```python
from build123d import *

# Parameters (mm, degrees)
SKETCH_1_W          = 57.5
SKETCH_1_H          = 46.5
EXTRUDE_1_DEPTH     = 3
SKETCH_2_R          = 1
CUT_EXTRUDE_1_DEPTH = 38.096158831
SKETCH_4_R          = 2.6
CUT_EXTRUDE_2_DEPTH = 0.8


with BuildPart() as part:
    # 草图1 → 凸台-拉伸1 (new body)
    with BuildSketch(Plane(origin=(0, 0, 0), x_dir=(1, 0, 0), z_dir=(0, 1, 0))):
        Rectangle(SKETCH_1_W, SKETCH_1_H)
    extrude(amount=EXTRUDE_1_DEPTH)

    # 草图2 → 切除-拉伸1 (cut, through all)
    with BuildSketch(Plane(origin=(0, 3, 0), x_dir=(1, 0, 0), z_dir=(0, 1, 0))):
        with Locations(Location((0, -15.1, 0), (0, 0, 270))):
            Circle(SKETCH_2_R)
        with Locations(Location((0, 15.1, 0), (0, 0, 270))):
            Circle(SKETCH_2_R)
    extrude(amount=-CUT_EXTRUDE_1_DEPTH, mode=Mode.SUBTRACT)

    # 草图4 → 切除-拉伸2 (cut)
    with BuildSketch(Plane.XZ):
        with Locations(Location((-20.75, 15.25, 0), (0, 0, 270))):
            Circle(SKETCH_4_R)
        with Locations(Location((20.75, 15.25, 0), (0, 0, 90))):
            Circle(SKETCH_4_R)
        with Locations(Location((-20.75, -15.25, 0), (0, 0, 90))):
            Circle(SKETCH_4_R)
        with Locations(Location((20.75, -15.25, 0), (0, 0, 270))):
            Circle(SKETCH_4_R)
    extrude(amount=-CUT_EXTRUDE_2_DEPTH, mode=Mode.SUBTRACT)


solid = part.part
```
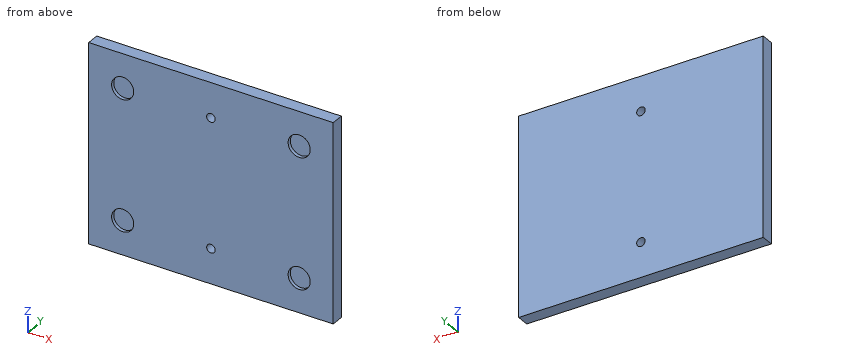
Input: part model. Units: mm. Frame: model coordinates. Coordinates: 2 decimals unless noted, no trailing zeros. Write each loop counter-clockwise with the first axis right and the second up, starting at its lowest first coordinate (ties: lowest second). Pieces come first, ordered by that corner, then holes. Notation, with made-up numbers: M -18,34.25 L 20,34.25 A21 cw 20,51.25 Z; hole C 5.5,9.5 d10. An arc over 180 degrees is marked long. Use one line per item in the form item = value.
Q1. Section D-D (z = 15.1). Return loops of the section in (x, y).
Answer below:
outline = M -28.75,0 L -23.35,0 L -23.35,0.8 L -18.15,0.8 L -18.15,0 L -1,0 L -1,3 L -28.75,3 Z; M 1,0 L 18.15,0 L 18.15,0.8 L 23.35,0.8 L 23.35,0 L 28.75,0 L 28.75,3 L 1,3 Z
Q2. First-contact query: pin 1 (1.6 mm diameter, centred on x = 0, z = -15.1, fed in from -Y); pin 2 (3 mm diameter, centred on x = 20.75, z = -15.25, fed in from -Y). Flat tips, straight axial feed; report the tip coordinate or a pass-through.
Answer below:
pin_1 = through
pin_2 = 0.8
Q3. Section C-C (x = 20.75). Return loops of the section in (y, z), plus the area to 3 significant figures.
Answer below:
outline = M 0,-23.25 L 3,-23.25 L 3,23.25 L 0,23.25 L 0,17.85 L 0.8,17.85 L 0.8,12.65 L 0,12.65 L 0,-12.65 L 0.8,-12.65 L 0.8,-17.85 L 0,-17.85 Z
area = 131 mm²
Q4. Section B-B (z = -15.5). Return loops of the section in (x, y), plus the area to 3 significant figures.
Answer below:
outline = M -28.75,0 L -23.34,0 L -23.34,0.8 L -18.16,0.8 L -18.16,0 L -0.92,0 L -0.92,3 L -28.75,3 Z; M 0.92,0 L 18.16,0 L 18.16,0.8 L 23.34,0.8 L 23.34,0 L 28.75,0 L 28.75,3 L 0.92,3 Z
area = 159 mm²
Q5. Material intervals for probe 1 along X at (y, z) = (0.4, 15.25); probe 2 along X at (y, z) = (1.45, -15.1); probe 3 along Z at (x, y) = (21, 0.25), sorted ascending. Write a range as from..to.
Answer below:
probe_1 = -28.75..-23.35, -18.15..-0.99, 0.99..18.15, 23.35..28.75
probe_2 = -28.75..-1, 1..28.75
probe_3 = -23.25..-17.84, -12.66..12.66, 17.84..23.25
Q6. Section A-A (x = 0). Return loops of the section in (y, z).
Answer below:
outline = M 0,-23.25 L 3,-23.25 L 3,-16.1 L 0,-16.1 Z; M 0,-14.1 L 3,-14.1 L 3,14.1 L 0,14.1 Z; M 0,16.1 L 3,16.1 L 3,23.25 L 0,23.25 Z
